from build123d import *

# Parameters (mm, degrees)
SKETCH1_W                      = 96
SKETCH1_H                      = 96
SKETCH1_R                      = 16.5
SKETCH1_R_2                    = 13.97
BOSS_EXTRUDE1_DEPTH            = 10
FILLET1_R                      = 20
M3_CLEARANCE_HOLE1_D           = 3.4
M3_CLEARANCE_HOLE1_CSINK_D     = 3.45
M3_CLEARANCE_HOLE1_CSINK_ANGLE = 90
CUT_EXTRUDE1_DEPTH             = 5
FILLET2_R                      = 3
CUT_EXTRUDE2_DEPTH             = 69.614867208


with BuildPart() as part:
    # Sketch1 → Boss-Extrude1 (new body)
    with BuildSketch(Plane(origin=(0, 0, 0), x_dir=(1, 0, 0), z_dir=(0, 1, 0))):
        Rectangle(SKETCH1_W, SKETCH1_H)
        with Locations(Location((-24, 24, 0), (0, 0, 270))):
            Circle(SKETCH1_R, mode=Mode.SUBTRACT)
        with Locations(Location((24, 24, 0), (0, 0, 90))):
            Circle(SKETCH1_R, mode=Mode.SUBTRACT)
        with Locations(Location((24, -24, 0), (0, 0, 270))):
            Circle(SKETCH1_R, mode=Mode.SUBTRACT)
        with Locations(Location((-24, -24, 0), (0, 0, 90))):
            Circle(SKETCH1_R, mode=Mode.SUBTRACT)
        with Locations(Location((0, 0, 0), (0, 0, 270))):
            Circle(SKETCH1_R_2, mode=Mode.SUBTRACT)
    extrude(amount=BOSS_EXTRUDE1_DEPTH)

    # Fillet1
    fillet1_edges = [part.edges().sort_by_distance(p)[0] for p in [
        (-48, 5, -48),
        (48, 5, -48),
        (48, 5, 48),
        (-48, 5, 48),
    ]]
    fillet(fillet1_edges, radius=FILLET1_R)

    # M3 Clearance Hole1 (through all)
    with Locations(Plane(origin=(-40, 0, 0), x_dir=(0, 0, -1), z_dir=(0, -1, 0))):
        with Locations((0, 0), (-40, 40), (0, 80), (40, 40)):
            CounterSinkHole(M3_CLEARANCE_HOLE1_D / 2, M3_CLEARANCE_HOLE1_CSINK_D / 2, counter_sink_angle=M3_CLEARANCE_HOLE1_CSINK_ANGLE)

    # Sketch7 → Cut-Extrude1 (cut)
    with BuildSketch(Plane.XZ):
        with BuildLine():
            Line((-9, 17.126136458), (9, 17.126136458))
            ThreePointArc((9, 17.126136458), (7.5, 24), (9, 30.873863542))
            Line((9, 30.873863542), (-9, 30.873863542))
            ThreePointArc((-9, 30.873863542), (-7.879361055, 27.51781182), (-7.5, 24))
            ThreePointArc((-7.5, 24), (-7.879361055, 20.48218818), (-9, 17.126136458))
        make_face()
        with BuildLine():
            ThreePointArc((9, -30.873863542), (7.5, -24), (9, -17.126136458))
            Line((9, -17.126136458), (-9, -17.126136458))
            ThreePointArc((-9, -17.126136458), (-7.879361055, -20.48218818), (-7.5, -24))
            ThreePointArc((-7.5, -24), (-7.879361055, -27.51781182), (-9, -30.873863542))
            Line((-9, -30.873863542), (9, -30.873863542))
        make_face()
    extrude(amount=-CUT_EXTRUDE1_DEPTH, mode=Mode.SUBTRACT)

    # Fillet2
    fillet2_edges = [part.edges().sort_by_distance(p)[0] for p in [
        (0, 0, 30.873863542),
        (0, 0, 17.126136458),
        (0, 0, -30.873863542),
        (0, 0, -17.126136458),
    ]]
    fillet(fillet2_edges, radius=FILLET2_R)

    # Sketch7_3 → Cut-Extrude2 (cut, through all)
    with BuildSketch(Plane.XZ):
        with BuildLine():
            Line((-17.126136458, -9), (-17.126136458, 9))
            ThreePointArc((-17.126136458, 9), (-24, 7.5), (-30.873863542, 9))
            Line((-30.873863542, 9), (-30.873863542, -9))
            ThreePointArc((-30.873863542, -9), (-24, -7.5), (-17.126136458, -9))
        make_face()
        with BuildLine():
            Line((30.873863542, -9), (30.873863542, 9))
            ThreePointArc((30.873863542, 9), (24, 7.5), (17.126136458, 9))
            Line((17.126136458, 9), (17.126136458, -9))
            ThreePointArc((17.126136458, -9), (24, -7.5), (30.873863542, -9))
        make_face()
    extrude(amount=-CUT_EXTRUDE2_DEPTH, mode=Mode.SUBTRACT)


solid = part.part
For this review, take the finished solid that the model builds, in its own axes (mm). A direction names the side the tool comes from. Give positions to 0.01 mm unless a question says otherwise; leave off trailing zeros. Loops run counter-clockwise (first coordinate to the right, second up) from the corner with the lowest first, then second, coordinate; pieces in that order, holes last.
Item 1: For line 1 along X through (y, z) = (5.25, 0); line 2 along X through (y, z) = (6.5, -24); line 3 along X through (y, z) = (7.25, -39), list the stretches that pass through material, from the lowest coordinate up.
Item 2: Take a section at A-A, the plane x = 24. State the section outline as (y, z) points, and give its area (3 significant figures).
Item 3: Insertion check: pin 1 (5 mm diameter, centred on x = 26, z = 37, fed in from -Y); pin 2 (4 mm diameter, centred on x = -4.5, z = 20.5, fed in from -Y); pin 3 (11 mm diameter, centred on x = -1, z = -26.5, fed in from -Y). Each pin has a flat end and moves straight along its axis. Give the tip position at first contact, or say it passes through.
Item 4: Take a section at B-B, the plane z = 0. State the section outline as (x, y) points (3 decimals), and give its area (3 significant figures).
Item 5: Draft analysis for pull direction Z (two halves, no side actions). For faces 4 (the flat face through (17.126, 5, 0)), 5 (the flat face through (-6, 0, -13)), 6 (the flat face through (0, 5, 48)), state which applies: +Z half, -Z half, draft (parallel to the pull), parting line (faces both ways), or undercut.
Item 6: Tool access review of faces 1 (the flat face through (0, 5, -48)), 2 (the flat face through (-17.126, 5, 0)), 3 (the cylindrical face through (0.151, 0.855, 16.224)): name each direction out of +Z, -Z, +X, -X, +Y, -Y from which nothing blocks a thin tool from reaching the whole face with its end or side.
Item 7: Take a section at D-D, the plane y = 7.25. State the section outline as (x, z) points, and give its area (3 significant figures).
Item 8: Take a section at C-C, the plane x = 0. Give the number of separate pieces and of enclosed holes in the cut face, and give its area (3 significant figures).
Calculated:
1. line 1: x = -48 to -41.7, -38.3 to -30.87, -17.13 to -13.97, 13.97 to 17.13, 30.87 to 38.3, 41.7 to 48
1. line 2: x = -48 to -40.5, -7.5 to 7.5, 40.5 to 48
1. line 3: x = -44.7 to -30.87, -17.13 to -1.37, 1.37 to 17.13, 30.87 to 44.7
2. outline: (0, -48) - (10, -48) - (10, -40.5) - (0, -40.5) - close; (0, 40.5) - (10, 40.5) - (10, 48) - (0, 48) - close
2. area: 150 mm2
3. pin 1: passes through
3. pin 2: stops at y = 5
3. pin 3: stops at y = 0.66
4. outline: (-48, 0) - (-41.725, 0) - (-41.7, 0.025) - (-41.7, 10) - (-48, 10) - close; (-38.3, 0.025) - (-38.275, 0) - (-30.874, 0) - (-30.874, 10) - (-38.3, 10) - close; (-17.126, 0) - (-13.97, 0) - (-13.97, 10) - (-17.126, 10) - close; (13.97, 0) - (17.126, 0) - (17.126, 10) - (13.97, 10) - close; (30.874, 0) - (38.275, 0) - (38.3, 0.025) - (38.3, 10) - (30.874, 10) - close; (41.7, 0.025) - (41.725, 0) - (48, 0) - (48, 10) - (41.7, 10) - close
4. area: 338 mm2
5. face 4: undercut
5. face 5: draft
5. face 6: +Z half
6. face 1: -Z, +X, -X, +Y, -Y
6. face 2: +Y, -Y
6. face 3: -Y
7. outline: (-48, -28) arc R20 ccw to (-28, -48) - (28, -48) arc R20 ccw to (48, -28) - (48, 28) arc R20 ccw to (28, 48) - (-28, 48) arc R20 ccw to (-48, 28) - close; hole circle Ø3.4 at (-40, 0); hole (-30.87, -9) arc R16.5 ccw (long way) to (-17.13, -9) - (-17.13, 9) arc R16.5 ccw (long way) to (-30.87, 9) - close; hole circle Ø27.94 at (0, 0); hole circle Ø3.4 at (0, -40); hole circle Ø3.4 at (0, 40); hole (17.13, -9) arc R16.5 ccw (long way) to (30.87, -9) - (30.87, 9) arc R16.5 ccw (long way) to (17.13, 9) - close; hole circle Ø3.4 at (40, 0)
7. area: 4,360 mm2
8. separate pieces: 4
8. enclosed holes: 0
8. area: 467 mm2
